Geometry: see drawing. Coordinates: mm, zero at the bounding-box minimum. A direction names the side the tool comes from. Give positions to 0.01 mm unless a question says otherwise; leave off trailing zeros. Write each loop counter-clockwise with the first axis right and the second up, starting at its lowest first coordinate (ties: lowest second). Pieces come first, ordered by that corner, then holes. Notation, with made-up numbers: (-20.5, 29) - (-4.5, 29) arc R9 ccw to (-4.5, 45) - close; hole circle Ø2 at (48, 49.25). An arc over 180 degrees is marked (long way). One line per question, with ' | ' between items. Start each with the question number.
(1) Section C-C, the plane y = 1. Return loops of the section in (x, z), plus the area to 3 significant figures.
(2) Section A-A, the plane x = 6.9. Return loops of the section in (y, z), plus the area to 3 significant figures.
(3) Section B-B, the plane z = 1.25. Return loops of the section in (x, y), plus the area to 3 significant figures.
(4) Section D-D, the plane x = 12.25. Return loops of the section in (y, z).
(5) Ray query, line 1 (Z direction, x = 6.9, y = 5.5); line 2 (Y direction, x = 5.75, z = 6.75); line 3 (Z direction, x = 1.5, y = 6). Return the intervals inside material, ascending. Write a range as [from, to].
(6) Pin query (flat end, axial travel): pin 1 (3 mm diameter, centred on y = 5.5, z = 3, fed in from +X); pin 2 (1.9 mm diameter, centred on x = 8, y = 4, fed in from -Z). Return the tip coordinate at first contact, or that it passes through.
(7) Draft query along X for the marked faces 4, 5 and 6. Return one class per face: +X half, -X half, draft (parallel to the pull), parting line (faces both ways), or undercut.
(8) Access query for the marked faces 1, 2 and 3. Directions: +Z, -Z, +X, -X, +Y, -Y. A direction counts if a zero-diameter tool reaches every point of the face in a straight line with its end or side. Return the directions, or none.
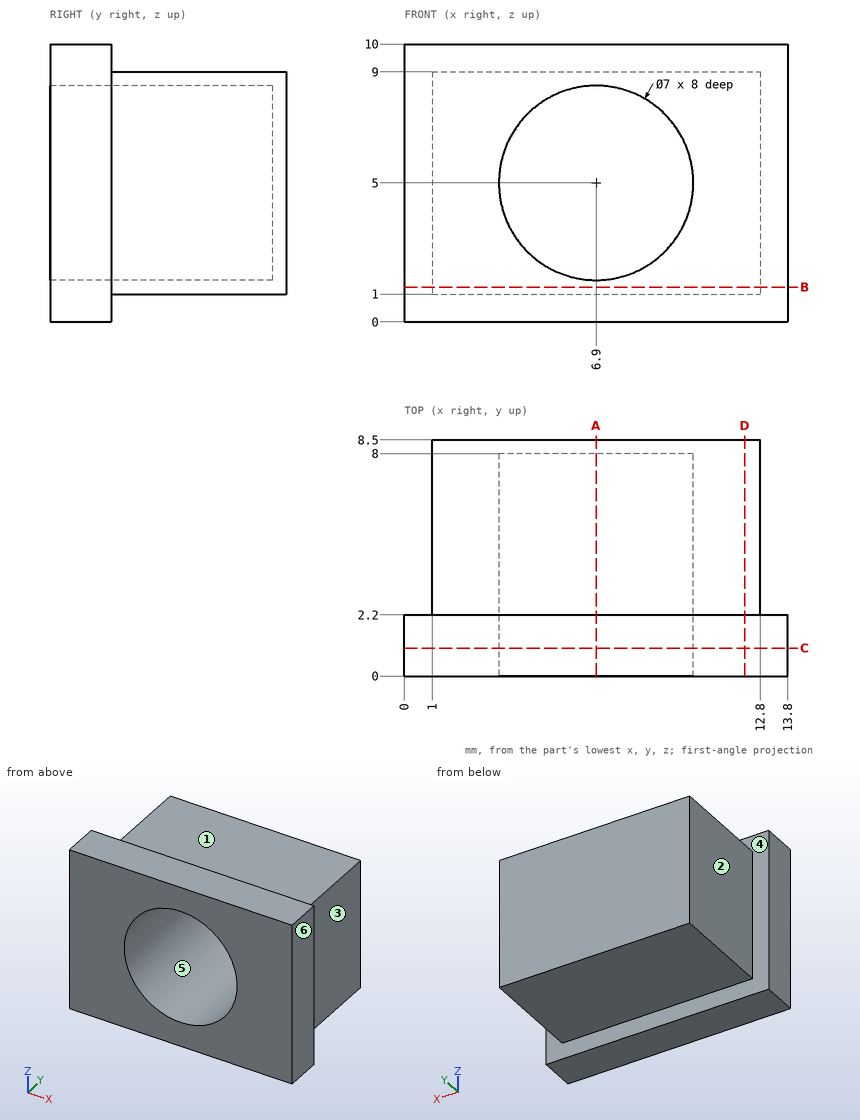
Check sheet entries:
1) outline: (0, 0) - (13.8, 0) - (13.8, 10) - (0, 10) - close; hole circle Ø7 at (6.9, 5) | area: 99.5 mm²
2) outline: (0, 0) - (2.2, 0) - (2.2, 1) - (8.5, 1) - (8.5, 9) - (2.2, 9) - (2.2, 10) - (0, 10) - (0, 8.5) - (8, 8.5) - (8, 1.5) - (0, 1.5) - close | area: 16.4 mm²
3) outline: (0, 0) - (13.8, 0) - (13.8, 2.2) - (12.8, 2.2) - (12.8, 8.5) - (1, 8.5) - (1, 2.2) - (0, 2.2) - close | area: 105 mm²
4) outline: (0, 0) - (2.2, 0) - (2.2, 1) - (8.5, 1) - (8.5, 9) - (2.2, 9) - (2.2, 10) - (0, 10) - close
5) line 1: [1, 1.5], [8.5, 9] | line 2: [8, 8.5] | line 3: [1, 9]
6) pin 1: x = 12.8 | pin 2: z = 1
7) face 4: draft | face 5: undercut | face 6: +X half
8) face 1: +Z, +X, -X, +Y | face 2: +Z, -Z, -X, +Y | face 3: +Z, -Z, +X, +Y
